Here's how the part is built. I have some questions about the finished solid (model axes, mm). A direction names the side the tool comes from. Give positions to 0.01 mm unless a question says otherwise; leave off trailing zeros. Loops run counter-clockwise (first coordinate to the right, second up) from the corner with the lowest first, then second, coordinate; pieces in that order, holes last. Notation, with made-up numbers: (33, 42) - (56, 42) arc R10 ccw to (56, 56) - close; hole circle Ø2 at (1.25, 70.25). An arc over 180 degrees is marked (long way). Return JSON: item names as keys, results as strings. Group by question number.
(1) If we section it at B-B (y = 3.75): Please give me the cut outline in (x, z), then the cut area to 3 significant figures.
(2) I need wall thicknesses on probe 1 along Y at (x, z) = (-12.5, -5.9); probe 2 along X at (y, z) = (1, 1.75); probe 3 along Y at (x, z) = (12.5, -2.95). Which ranges of each line are inside material? Lowest first, please. Write a range as [from, to].
(3) On a 3-axis mill with a long thin cutter (end or side, diameter ignored), from which of +Z, -Z, +X, -X, +Y, -Y can I reach the whole of each face in a straight line? I mean faces 1 (the cylindrical face through (-12.976, 8.385, 9.26)), 2 (the flat face through (0, 9, 10)), 3 (the flat face through (0, 4, 5)). Say none if no direction works.
(4) If we section it at A-A (z = -1): Please give me the cut outline in (x, y).
(5) For P1, Ø1.3, axis at x = -13, y = -1, coming from the +Z side; P2, Ø1, axis at x = 12.5, y = -9, coming from the +Z side; P3, Ø1.5, axis at x = -1, z = -3, coming from the -Y side, each with a flat end and sliding along its axis, tell me the tip position at first contact or that it passes through.
(6) If we mould it in two halves opening along X, with no side actions, what happens to faces 4 (the flat face through (15, 2, -2)), 5 (the flat face through (0, -10, -9)), 6 (the flat face through (12.5, 1.3, 1))? For each: released by +X, released by -X, zero draft, split by the parting line, or undercut.
(7) If we section it at C-C (x = 1.5): Please give me the cut outline in (y, z).
(8) If we section it at D-D (y = -3.75): Please give me the cut outline in (x, z).
```python
from build123d import *

# Parameters (mm, degrees)
SKETCH_W        = 30
SKETCH_H        = 20
PAD_DEPTH       = 10
SKETCH001_W     = 30
SKETCH001_H     = 2.5
POCKET_DEPTH    = 17.5
SKETCH002_W     = 30
SKETCH002_H     = 2.5
POCKET001_DEPTH = 15
SKETCH003_W     = 30
SKETCH003_H     = 2.5
POCKET002_DEPTH = 12.5
SKETCH004_W     = 30
SKETCH004_H     = 2.5
POCKET003_DEPTH = 10
SKETCH005_W     = 30
SKETCH005_H     = 2.5
POCKET004_DEPTH = 7.5
SKETCH006_W     = 30
SKETCH006_H     = 2.5
POCKET005_DEPTH = 5
SKETCH007_W     = 30
SKETCH007_H     = 2.5
POCKET006_DEPTH = 2.5
SKETCH008_R     = 0.6
POCKET007_DEPTH = 1.5
SKETCH009_R     = 0.6
POCKET008_DEPTH = 1.5
SKETCH010_R     = 0.6
POCKET009_DEPTH = 1.5
SKETCH011_R     = 0.6
POCKET010_DEPTH = 1.5
SKETCH012_R     = 0.6
POCKET011_DEPTH = 1.5
SKETCH013_R     = 0.6
POCKET012_DEPTH = 1.5
SKETCH014_R     = 0.6
POCKET013_DEPTH = 1.5
SKETCH015_R     = 0.6
POCKET014_DEPTH = 1.5


with BuildPart() as part:
    # Sketch → Pad (new body, symmetric)
    with BuildSketch(Plane.XY):
        Rectangle(SKETCH_W, SKETCH_H)
    extrude(amount=PAD_DEPTH, both=True)

    # Sketch001 → Pocket (cut)
    with BuildSketch(Plane.XY.offset(10)):
        with Locations((0, -8.75)):
            Rectangle(SKETCH001_W, SKETCH001_H)
    extrude(amount=-POCKET_DEPTH, mode=Mode.SUBTRACT)

    # Sketch002 → Pocket001 (cut)
    with BuildSketch(Plane.XY.offset(10)):
        with Locations((0, -6.25)):
            Rectangle(SKETCH002_W, SKETCH002_H)
    extrude(amount=-POCKET001_DEPTH, mode=Mode.SUBTRACT)

    # Sketch003 → Pocket002 (cut)
    with BuildSketch(Plane.XY.offset(10)):
        with Locations((0, -3.75)):
            Rectangle(SKETCH003_W, SKETCH003_H)
    extrude(amount=-POCKET002_DEPTH, mode=Mode.SUBTRACT)

    # Sketch004 → Pocket003 (cut)
    with BuildSketch(Plane.XY.offset(10)):
        with Locations((0, -1.25)):
            Rectangle(SKETCH004_W, SKETCH004_H)
    extrude(amount=-POCKET003_DEPTH, mode=Mode.SUBTRACT)

    # Sketch005 → Pocket004 (cut)
    with BuildSketch(Plane.XY.offset(10)):
        with Locations((0, 1.25)):
            Rectangle(SKETCH005_W, SKETCH005_H)
    extrude(amount=-POCKET004_DEPTH, mode=Mode.SUBTRACT)

    # Sketch006 → Pocket005 (cut)
    with BuildSketch(Plane.XY.offset(10)):
        with Locations((0, 3.75)):
            Rectangle(SKETCH006_W, SKETCH006_H)
    extrude(amount=-POCKET005_DEPTH, mode=Mode.SUBTRACT)

    # Sketch007 → Pocket006 (cut)
    with BuildSketch(Plane.XY.offset(10)):
        with Locations((0, 6.25)):
            Rectangle(SKETCH007_W, SKETCH007_H)
    extrude(amount=-POCKET006_DEPTH, mode=Mode.SUBTRACT)

    # Sketch008 → Pocket007 (cut)
    with BuildSketch(Plane.XY.offset(-7.5)):
        with Locations((-12.5, -8.75)):
            Circle(SKETCH008_R)
        with Locations((12.5, -8.75)):
            Circle(SKETCH008_R)
    extrude(amount=-POCKET007_DEPTH, mode=Mode.SUBTRACT)

    # Sketch009 → Pocket008 (cut)
    with BuildSketch(Plane.XY.offset(-5)):
        with Locations((-12.5, -6.25)):
            Circle(SKETCH009_R)
        with Locations((12.5, -6.25)):
            Circle(SKETCH009_R)
    extrude(amount=-POCKET008_DEPTH, mode=Mode.SUBTRACT)

    # Sketch010 → Pocket009 (cut)
    with BuildSketch(Plane.XY.offset(-2.5)):
        with Locations((-12.5, -3.75)):
            Circle(SKETCH010_R)
        with Locations((12.5, -3.75)):
            Circle(SKETCH010_R)
    extrude(amount=-POCKET009_DEPTH, mode=Mode.SUBTRACT)

    # Sketch011 → Pocket010 (cut)
    with BuildSketch(Plane.XY):
        with Locations((-12.5, -1.25)):
            Circle(SKETCH011_R)
        with Locations((12.5, -1.25)):
            Circle(SKETCH011_R)
    extrude(amount=-POCKET010_DEPTH, mode=Mode.SUBTRACT)

    # Sketch012 → Pocket011 (cut)
    with BuildSketch(Plane.XY.offset(2.5)):
        with Locations((-12.5, 1.25)):
            Circle(SKETCH012_R)
        with Locations((12.5, 1.25)):
            Circle(SKETCH012_R)
    extrude(amount=-POCKET011_DEPTH, mode=Mode.SUBTRACT)

    # Sketch013 → Pocket012 (cut)
    with BuildSketch(Plane.XY.offset(5)):
        with Locations((-12.5, 3.75)):
            Circle(SKETCH013_R)
        with Locations((12.5, 3.75)):
            Circle(SKETCH013_R)
    extrude(amount=-POCKET012_DEPTH, mode=Mode.SUBTRACT)

    # Sketch014 → Pocket013 (cut)
    with BuildSketch(Plane.XY.offset(7.5)):
        with Locations((-12.5, 6.25)):
            Circle(SKETCH014_R)
        with Locations((12.5, 6.25)):
            Circle(SKETCH014_R)
    extrude(amount=-POCKET013_DEPTH, mode=Mode.SUBTRACT)

    # Sketch015 → Pocket014 (cut)
    with BuildSketch(Plane.XY.offset(10)):
        with Locations((-12.5, 8.75)):
            Circle(SKETCH015_R)
        with Locations((12.5, 8.75)):
            Circle(SKETCH015_R)
    extrude(amount=-POCKET014_DEPTH, mode=Mode.SUBTRACT)


solid = part.part
```
Values:
{
 "1": {"outline": "(-15, -10) - (15, -10) - (15, 5) - (13.1, 5) - (13.1, 3.5) - (11.9, 3.5) - (11.9, 5) - (-11.9, 5) - (-11.9, 3.5) - (-13.1, 3.5) - (-13.1, 5) - (-15, 5) - close", "area": "446 mm2"},
 "2": {"probe 1": "[-7.5, -6.85], [-5.65, 10]", "probe 2": "[-15, -13.05], [-11.95, 11.95], [13.05, 15]", "probe 3": "[-5, -4.35], [-3.15, 10]"},
 "3": {"face 1": "+Z", "face 2": "+Z, +X, -X, +Y, -Y", "face 3": "+Z, +X, -X, -Y"},
 "4": {"outline": "(-15, -2.5) - (15, -2.5) - (15, 10) - (-15, 10) - close; hole circle Ø1.2 at (-12.5, -1.25); hole circle Ø1.2 at (12.5, -1.25)"},
 "5": {"P1": "z = 0", "P2": "z = -7.5", "P3": "y = -5"},
 "6": {"face 4": "released by +X", "face 5": "zero draft", "face 6": "undercut"},
 "7": {"outline": "(-10, -10) - (10, -10) - (10, 10) - (7.5, 10) - (7.5, 7.5) - (5, 7.5) - (5, 5) - (2.5, 5) - (2.5, 2.5) - (0, 2.5) - (0, 0) - (-2.5, 0) - (-2.5, -2.5) - (-5, -2.5) - (-5, -5) - (-7.5, -5) - (-7.5, -7.5) - (-10, -7.5) - close"},
 "8": {"outline": "(-15, -10) - (15, -10) - (15, -2.5) - (13.1, -2.5) - (13.1, -4) - (11.9, -4) - (11.9, -2.5) - (-11.9, -2.5) - (-11.9, -4) - (-13.1, -4) - (-13.1, -2.5) - (-15, -2.5) - close"}
}
